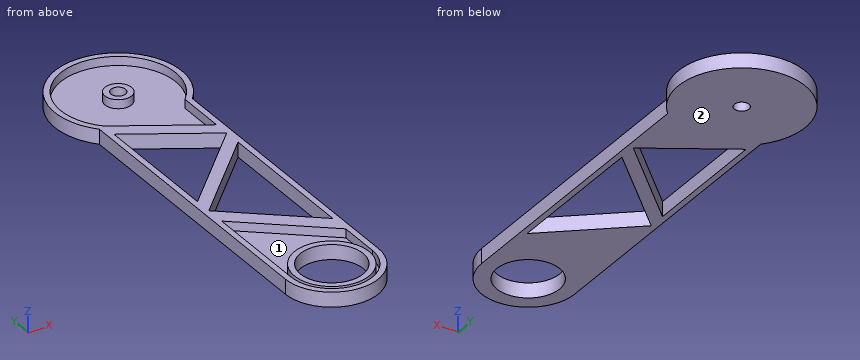
from build123d import *

# Parameters (mm, degrees)
SKETCH1_R           = 13.5
SKETCH1_R_2         = 3.175
BOSS_EXTRUDE1_DEPTH = 6.35
SHELL1_T            = -2.54
BOSS_EXTRUDE2_DEPTH = 3.81
BOSS_EXTRUDE3_DEPTH = 3.81
CUT_EXTRUDE1_DEPTH  = 141.327742832


with BuildPart() as part:
    # Sketch1 → Boss-Extrude1 (new body)
    with BuildSketch(Plane.XY):
        with BuildLine():
            Line((-11.394392523, 89.748598131), (-11.394392523, -35.251401869))
            ThreePointArc((-11.394392523, -35.251401869), (8.605607477, -55.251401869), (28.605607477, -35.251401869))
            Line((28.605607477, -35.251401869), (28.605607477, 89.748598131))
            ThreePointArc((28.605607477, 89.748598131), (8.605607477, 135.605580593), (-11.394392523, 89.748598131))
        make_face()
        with Locations((8.605607477, -35.251401869)):
            Circle(SKETCH1_R, mode=Mode.SUBTRACT)
        with Locations((8.605607477, 108.315703391)):
            Circle(SKETCH1_R_2, mode=Mode.SUBTRACT)
    extrude(amount=BOSS_EXTRUDE1_DEPTH)

    # Shell1
    shell1_openings = [part.faces().sort_by_distance(p)[0] for p in [
        (8.605607477, 50.282735683, 6.35),
    ]]
    offset(amount=SHELL1_T, openings=shell1_openings, kind=Kind.INTERSECTION)

    # Sketch2 → Boss-Extrude2 (add)
    with BuildSketch(Plane.XY.offset(6.35)):
        Polygon((-8.854392523, 27.76139222), (26.065607477, 62.68139222), (26.065607477, 55.06139222), (-8.854392523, 20.14139222), align=None)
    extrude(amount=-BOSS_EXTRUDE2_DEPTH)

    # Sketch3 → Boss-Extrude3 (add)
    with BuildSketch(Plane.XY.offset(2.54)):
        Polygon((26.065607477, 62.68139222), (-8.854392523, 83.913349477), (-8.854392523, 90.774186309), (26.065607477, 69.542229051), align=None)
        Polygon((-8.854392523, 20.14139222), (26.065607477, -8.685765345), (26.065607477, -17.33689372), (-8.854392523, 11.490263845), align=None)
    extrude(amount=BOSS_EXTRUDE3_DEPTH)

    # Sketch4 → Cut-Extrude1 (cut, through all)
    with BuildSketch(Plane.XY.offset(2.54)):
        Polygon((-8.854392523, 27.76139222), (26.065607477, 62.68139222), (-8.854392523, 83.913349477), align=None)
        Polygon((-8.854392523, 20.14139222), (26.065607477, -8.685765345), (26.065607477, 55.06139222), align=None)
    extrude(amount=-CUT_EXTRUDE1_DEPTH, mode=Mode.SUBTRACT)


solid = part.part
Source: CAD feature listing. Evaluate the final solid. Frame: model axes, mm. Face numbers are marked on the shaded views. Give positions to 0.01 mm unless a question says otherwise; leave off trailing zeros. Loops run counter-clockwise (first coordinate to the right, second up) from the corner with the lowest first, then second, coordinate; pieces in that order, holes last. Notation, with made-up numbers: (-16.75, 26.5) -> (27.25, 26.5) arc R32 ccw to (27.25, 64.5) -> close; hole circle Ø2 at (72.25, 75). An arc over 180 degrees is marked (long way). Use a Markdown table: item, result. Add a question column.
1) Line query: line 1 along X through (y, z) = (108, 0.75); line 2 along X through (y, z) = (48, 2); line 3 along Y through (x, z) = (0, 2.5). Output: solid intervals per line, ascending. Write a range as [from, to].
2) First-contact query: pin 1 (3 mm diameter, centred on y = 10, z = 4.5, fed in from -X); pin 2 (1.1 mm diameter, centred on y = -7.5, z = 5.5, fed in from +X); pin 3 (12 mm diameter, centred on x = 9.5, y = 83, fed in from +Z); pin 4 (15 mm diameter, centred on x = 15, y = 90, fed in from +Z). Flat tips, straight axial feed; report the tip coordinate or a pass-through.
3) Section query A-A, the plane z = 4.5. Count the separate pieces of the cut face and the enclosed holes in it, then the cut area to 3 significant figures.
4) Section query C-C, the plane y = 33.5. Return the cut outline in (x, z), then the cut area to 3 significant figures.
5) Section query B-B, the plane y = 59.5. Return the cut outline in (x, z).
6) Section query D-D, the plane x = -13.5. Return the cut outline in (y, z).
7) Pull-direction query (X, two-part tool) for the marked faces 1 and 2; classes: +X half, -X half, draft (parallel to the pull), parting line (faces both ways), or undercut.
Numbers:
| question | item | result |
|---|---|---|
| 1 | line 1 | x = [-18.68, 5.45], [11.76, 35.89] |
| 1 | line 2 | x = [-11.39, -8.85], [11.38, 19], [26.07, 28.61] |
| 1 | line 3 | y = [-53.31, -45.65], [-24.85, 12.83], [29, 36.62], [78.53, 134.21] |
| 2 | pin 1 | stops at x = -11.39 |
| 2 | pin 2 | stops at x = 28.61 |
| 2 | pin 3 | stops at z = 6.35 |
| 2 | pin 4 | stops at z = 2.54 |
| 3 | separate pieces | 3 |
| 3 | enclosed holes | 6 |
| 3 | area | 2,210 mm2 |
| 4 | outline | (-11.39, 0) -> (-8.85, 0) -> (-8.85, 6.35) -> (-11.39, 6.35) -> close; (-3.12, 0) -> (4.5, 0) -> (4.5, 6.35) -> (-3.12, 6.35) -> close; (26.07, 0) -> (28.61, 0) -> (28.61, 6.35) -> (26.07, 6.35) -> close |
| 4 | area | 80.6 mm2 |
| 5 | outline | (-11.39, 0) -> (-8.85, 0) -> (-8.85, 6.35) -> (-11.39, 6.35) -> close; (22.88, 0) -> (28.61, 0) -> (28.61, 6.35) -> (22.88, 6.35) -> close |
| 6 | outline | (92.31, 0) -> (124.32, 0) -> (124.32, 6.35) -> (119.45, 6.35) -> (119.45, 2.54) -> (97.18, 2.54) -> (97.18, 6.35) -> (92.31, 6.35) -> close |
| 7 | face 1 | undercut |
| 7 | face 2 | draft |
